For this review, use the dimensioned drawing (mm, ordinates from the lowest corner) and the shaded views. Coordinates: 2 decimals unless noted, no trailing zeros. Loops run counter-clockwise (first coordinate to the right, second up) from the corner with the lowest first, then second, coordinate; pieces in that order, holes last.
1. Take a section at A-A, the plane y = 2.5. State the section outline as (x, z) points, then the cut area to 3 significant figures.
2. Clearance check with flat-ended pins moving along their axes: P1, Ø1.5, axis at x = 1, y = 7, coming from the +Z side; P2, Ø1.8, axis at y = 2.5, z = 2.5, coming from the +X side. State where each tip first meets the part, or that it passes through.
3. Take a section at B-B, the plane z = 2.5. Count the separate pieces of the cut face and the enclosed holes in it, then the cut area to 3 significant figures.
4. Take a section at D-D, the plane y = 10.5. State the section outline as (x, z) points.
5. Mouldability with a two-part tool opening along Z and no side actions: class the marked faces 1, 2 and 3 as pulls with the +Z half, pulls with the -Z half, needs draft (parallel to the pull), parting line crosses it, or undercut.
6. To check wall thickness, follow probe 1 along Y at (x, z) = (3.1, 2.5); probe 2 along Y at (x, z) = (2.75, 1.85); probe 3 along Z at (x, y) = (3.05, 2.25). State the ranges of each line that lie inside material, in increasing order.
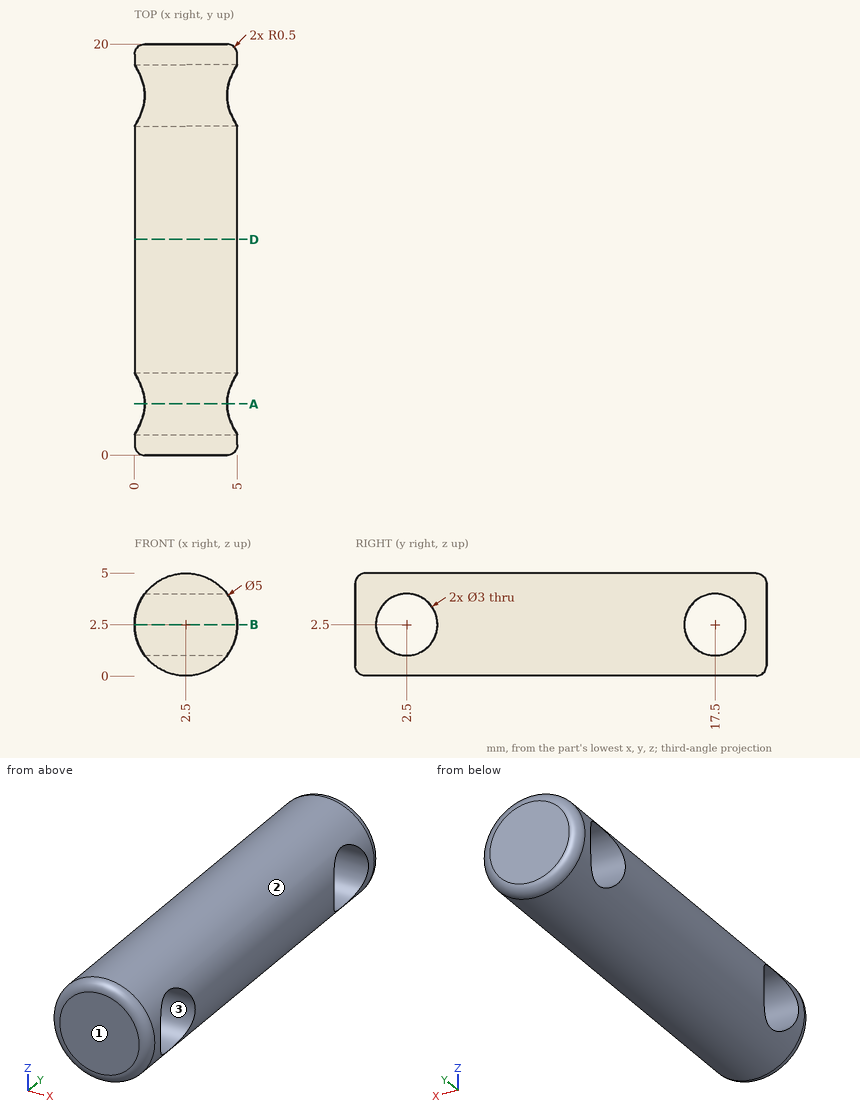
Results list:
1. outline: (0.5, 1) arc R2.5 ccw to (4.5, 1) - close; (0.5, 4) - (4.5, 4) arc R2.5 ccw to start
1. area: 5.59 mm2
2. P1: stops at z = 4.88
2. P2: passes through
3. separate pieces: 3
3. enclosed holes: 0
3. area: 69.8 mm2
4. outline: circle Ø5 at (2.5, 2.5)
5. face 1: needs draft
5. face 2: parting line crosses it
5. face 3: undercut
6. probe 1: y = 0 to 1, 4 to 16, 19 to 20
6. probe 2: y = 0 to 1.15, 3.85 to 16.15, 18.85 to 20
6. probe 3: z = 0.06 to 1.02, 3.98 to 4.94
